from build123d import *

# Parameters (mm, degrees)
F1_W           = 76.2
F1_H           = 76.2
F1_W_2         = 63.5
F1_H_2         = 63.5
F3_W           = 76.2
F3_H           = 76.2
F3_W_2         = 63.5
F3_H_2         = 63.5
F4_DEPTH       = 802.767
F4_DEPTH_BACK  = 802.767
F5_W           = 1757.934
F5_H           = 2.667
F6_DEPTH       = 660.4
F6_DEPTH_BACK  = 660.4
F7_W           = 19.05
F7_H           = 19.05
F8_DEPTH       = 793.75
F9_W           = 6.35
F9_H           = 25.4
F10_REACH      = 496.0827207226
F11_R          = 11.1125
F12_DEPTH      = 104.268
F13_R          = 9.525
F14_DEPTH      = 76.2
F15_R          = 6.35
F16_DEPTH      = 177.8
F16_DEPTH_BACK = 177.8


# Not quite as in the source:
# - an extrude ends at something that could not be found from the text; its depth is read off the source's solid


with BuildPart() as f2:
    # F2: sweep along a path in F0
    with BuildLine(Plane.XZ) as f2_path:
        Line((-878.967, 660.4), (878.967, 660.4))
        Line((878.967, 660.4), (878.967, -660.4))
        Line((878.967, -660.4), (-878.967, -660.4))
        Line((-878.967, -660.4), (-878.967, 660.4))
    # F1 (on Top) → F2 (sweep)
    with BuildSketch(Plane.XY):
        with Locations((-840.867, -38.1)):
            Rectangle(F1_W, F1_H)
        with Locations((-840.867, -38.1)):
            Rectangle(F1_W_2, F1_H_2, mode=Mode.SUBTRACT)
    sweep(path=f2_path.line, transition=Transition.RIGHT)

    # F3 (on Right) → F4 (join, two sides)
    with BuildSketch(Plane.YZ) as f4_sk:
        with Locations((-38.1, 215.9)):
            Rectangle(F3_W, F3_H)
        with Locations((-38.1, 215.9)):
            Rectangle(F3_W_2, F3_H_2, mode=Mode.SUBTRACT)
        with Locations((-38.1, -215.9)):
            Rectangle(F3_W, F3_H)
        with Locations((-38.1, -215.9)):
            Rectangle(F3_W_2, F3_H_2, mode=Mode.SUBTRACT)
    extrude(amount=-F4_DEPTH)
    extrude(f4_sk.sketch, amount=F4_DEPTH_BACK)

    # F5 (on Top) → F6 (join, two sides)
    with BuildSketch(Plane.XY) as f6_sk:
        with Locations((0, -77.5335)):
            Rectangle(F5_W, F5_H)
    extrude(amount=F6_DEPTH)
    extrude(f6_sk.sketch, amount=-F6_DEPTH_BACK)

    # F7 (on Right) → F8 (join, symmetric)
    with BuildSketch(Plane.YZ):
        Polygon((-78.867, 190.5), (-78.867, 215.9), (-102.5499750297, 215.9), (-104.267, 215.9), (-104.267, 190.5), align=None)
        with Locations((-91.567, 203.2)):
            Rectangle(F7_W, F7_H, mode=Mode.SUBTRACT)
        Polygon((-104.267, 215.9), (-102.5499750297, 215.9), (-78.867, 239.5829750297), (-78.867, 241.3), align=None)
    extrude(amount=F8_DEPTH, both=True)

    f10_end = Plane(origin=(0, -90.7084875148, 227.7414875149), x_dir=(0, 0.7071067812, 0.7071067812), z_dir=(0, 0.7071067812, -0.7071067812))
    # F9 (on face) → F10 (join, up to a plane its end follows)
    with BuildSketch(Plane(origin=(0, 0, 190.5000000001), x_dir=(1, 0, 0), z_dir=(0, 0, -1))):
        with Locations((790.575, 91.567)):
            Rectangle(F9_W, F9_H)
        with Locations((-790.575, 91.567)):
            Rectangle(F9_W, F9_H)
    f10_long = extrude(amount=-F10_REACH, mode=Mode.PRIVATE)
    add(split(f10_long, bisect_by=f10_end, keep=Keep.TOP, mode=Mode.PRIVATE))

    # F11 (on Front) → F12 (cut, through all)
    with BuildSketch(Plane.XZ):
        with Locations((-840.867, -76.2)):
            Circle(F11_R)
        with Locations((-840.867, -508)):
            Circle(F11_R)
        with Locations((-840.867, 76.2000000001)):
            Circle(F11_R)
        with Locations((-840.867, -355.6)):
            Circle(F11_R)
        with Locations((-840.867, 406.4)):
            Circle(F11_R)
        with Locations((-840.867, 558.8)):
            Circle(F11_R)
        with Locations((840.867, 558.8)):
            Circle(F11_R)
        with Locations((840.867, 406.4)):
            Circle(F11_R)
        with Locations((840.867, 76.2000000001)):
            Circle(F11_R)
        with Locations((840.867, -76.2)):
            Circle(F11_R)
        with Locations((840.867, -355.6)):
            Circle(F11_R)
        with Locations((840.867, -508)):
            Circle(F11_R)
    extrude(amount=F12_DEPTH, mode=Mode.SUBTRACT)

    # F13 (on face) → F14 (cut, through all)
    with BuildSketch(Plane.XY.offset(254)):
        with Locations((-726.567, -38.1)):
            Circle(F13_R)
        with Locations((726.567, -38.1)):
            Circle(F13_R)
    extrude(amount=-F14_DEPTH, mode=Mode.SUBTRACT)

    # F15 (on Top) → F16 (join, two sides)
    with BuildSketch(Plane.XY) as f16_sk:
        with Locations((-650.367, -12.7)):
            Circle(F15_R)
    extrude(amount=F16_DEPTH)
    extrude(f16_sk.sketch, amount=-F16_DEPTH_BACK)


solid = f2.part
For this review, take the finished solid that the model builds, in its own axes (mm). A direction names the side the tool comes from. Give positions to 0.01 mm unless a question says otherwise; leave off trailing zeros. Put each result on its own line as item: value. Start each with the question number.
(1) Add section A-A, the plane x = 579. Give the number of separate pieces and of enclosed holes in the cut face, then the cut area to 3 significant figures.
(2) The part is to be moulded in two halves that separate along Z. For faces 4 (the flat face through (4, -69.85, -633)), 5 (the flat face through (-12, -39, -660.4)), 6 (the flat face through (-12, -39, 660.4)), say which applies: +Z half, -Z half, draft (parallel to the pull), parting line (faces both ways), or undercut.
(3) Wall thickness on L1, parallel to X at y = -72, z = 558.8; L2, parallel to X at y = -60, z = 361; L3, parallel to Z at x = 86.5, y = -74.5: over which ranges is each line inside the solid? List them lowest first.
(4) Machinability: for faces 1 (the flat face through (-878.967, -40, 9)), 2 (the flat face through (11, -39, 584.2)), 3 (the flat face through (12, -39, 654.05)), which of the approach directions +Z, -Z, +X, -X, +Y, -Y give a long, thin tool a straight path to every point of the face, cutting with its end or side? Answer none if there is none.
(5) For pin 1 (5 mm diameter, centred on x = -518.5, z = 136.5, fed in from -Y); pin 2 (18 mm diameter, centred on x = 840.867, z = 406.4, fed in from -Y); pin 3 (12 mm diameter, centred on x = 685.5, z = -446.5, fed in from +Y); pin 4 (12.5 mm diameter, centred on x = 66.5, y = -96, fed in from -Z), all flat-tipped, find the tip position at first contact; note any pin that passes through.
Result:
1. separate pieces: 1
1. enclosed holes: 6
1. area: 10,900 mm^2
2. face 4: undercut
2. face 5: -Z half
2. face 6: +Z half
3. L1: x = -878.97 to -851.98, -829.75 to -802.77, 802.77 to 829.75, 851.98 to 878.97
3. L2: x = -878.97 to -872.62, -809.12 to -802.77, 802.77 to 809.12, 872.62 to 878.97
3. L3: z = -660.4 to -584.2, -254 to -177.8, 177.8 to 254, 584.2 to 660.4
4. face 1: +Z, -Z, -X, +Y, -Y
4. face 2: +Y
4. face 3: none
5. pin 1: stops at y = -78.87
5. pin 2: passes through
5. pin 3: stops at y = -76.2
5. pin 4: stops at z = 190.5
